Can you work these out from the drawing? Everything is in mm from the part's minimum corner. A direction names the side the tool comes from. Round coordinates to 2 decimals unless told otherwise and drop trailing zeros. Write each loop counter-clockwise with the first axis right and the second up, starting at its lowest first coordinate (ties: lowest second). Pieces come first, ordered by that corner, then holes. Notation, with made-up numbers: M -33,-20 L -21,-20 A28 cw -21,-2 Z; hole C 36,28 d10. An arc over 180 degrees is marked long. Use a Markdown table: item, result. Add a question column.
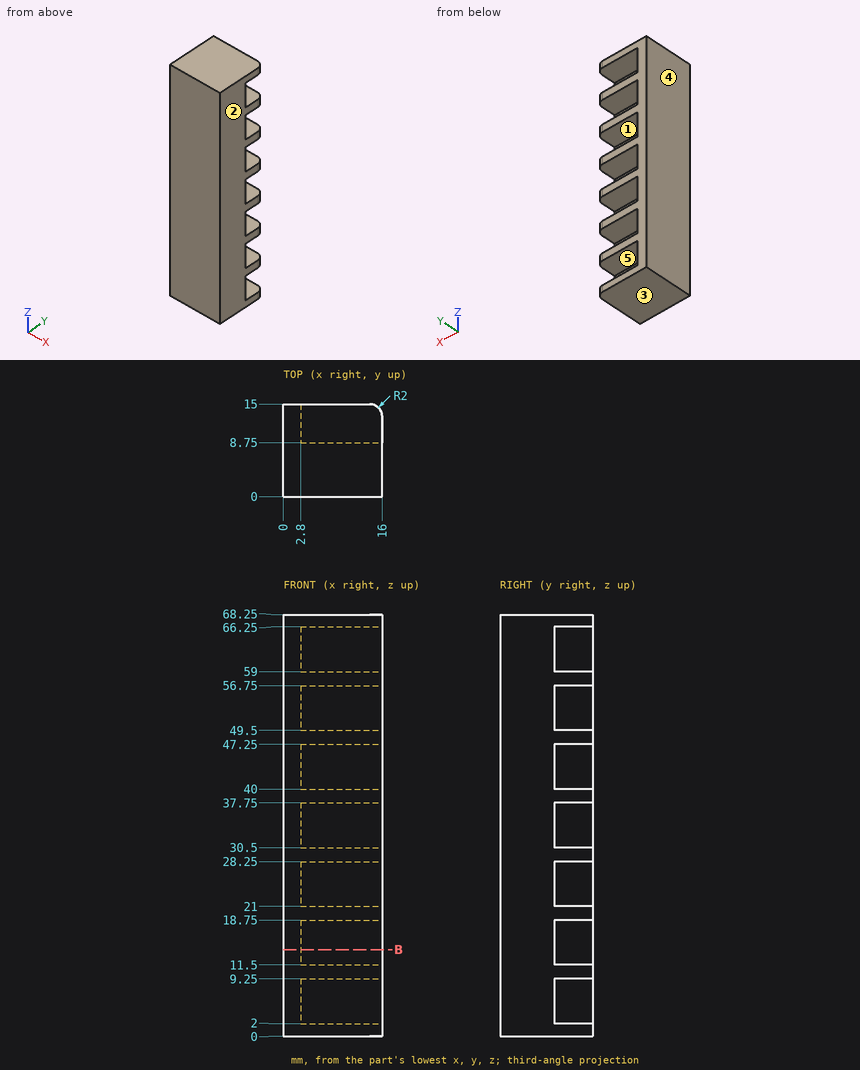
Item 1: If we mould it in two halves opening along Z, with no side actions, what happens to the marked faces 1, 2 and 3? For each: +Z half, -Z half, draft (parallel to the pull), parting line (faces both ways), or undercut.
Item 2: Imagine slicing it at B-B on z = 14. List the corners of the cut face in (x, y) for me, plus the area to 4 significant figures.
Item 3: For pin 1 Ø5 at (y, z) = (12.5, 24.5) entering from +X; pin 2 Ø2 at (x, z) = (7, 44) entering from +Y, each with a flat end and sliding along its axis, tell me the tip position at first contact or that it passes through.
Item 4: I need wall thicknesses on probe 1 along X at (y, z) = (13.5, 6); probe 2 along Y at (x, z) = (5.75, 9). Which ranges of each line are inside material? Lowest first, please. Write a range as from..to.
Item 5: On a 3-axis mill with a long thin cutter (end or side, diameter ignored), from which of +Z, -Z, +X, -X, +Y, -Y can I reach the whole of each face in a straight line? I mean the marked faces 4 and 5. Say none if no direction works.
The answers:
| question | item | result |
|---|---|---|
| 1 | face 1 | undercut |
| 1 | face 2 | draft |
| 1 | face 3 | -Z half |
| 2 | outline | M 0,0 L 16,0 L 16,8.75 L 2.8,8.75 L 2.8,15 L 0,15 Z |
| 2 | area | 157.5 mm² |
| 3 | pin 1 | x = 2.8 |
| 3 | pin 2 | y = 8.75 |
| 4 | probe 1 | 0..2.8 |
| 4 | probe 2 | 0..8.75 |
| 5 | face 4 | +Z, -Z, -X, +Y, -Y |
| 5 | face 5 | +X, +Y |
